Geometry check sheet. Reference: drawing and pictorial views, mm from the part's lowest x, y, z. A direction names the side the tool comes from. Round coordinates to 2 decimals unless told otherwise and drop trailing zeros. Loops run counter-clockwise (first coordinate to the right, second up) from the corner with the lowest first, then second, coordinate; pieces in that order, holes last. Notation, with made-up numbers: (-16.5, 36) - (24.5, 36) arc R18 cw to (24.5, 67) - close; hole circle Ø9 at (16.5, 19). An arc over 180 degrees is marked (long way). Return JSON: item names as keys, results as strings.
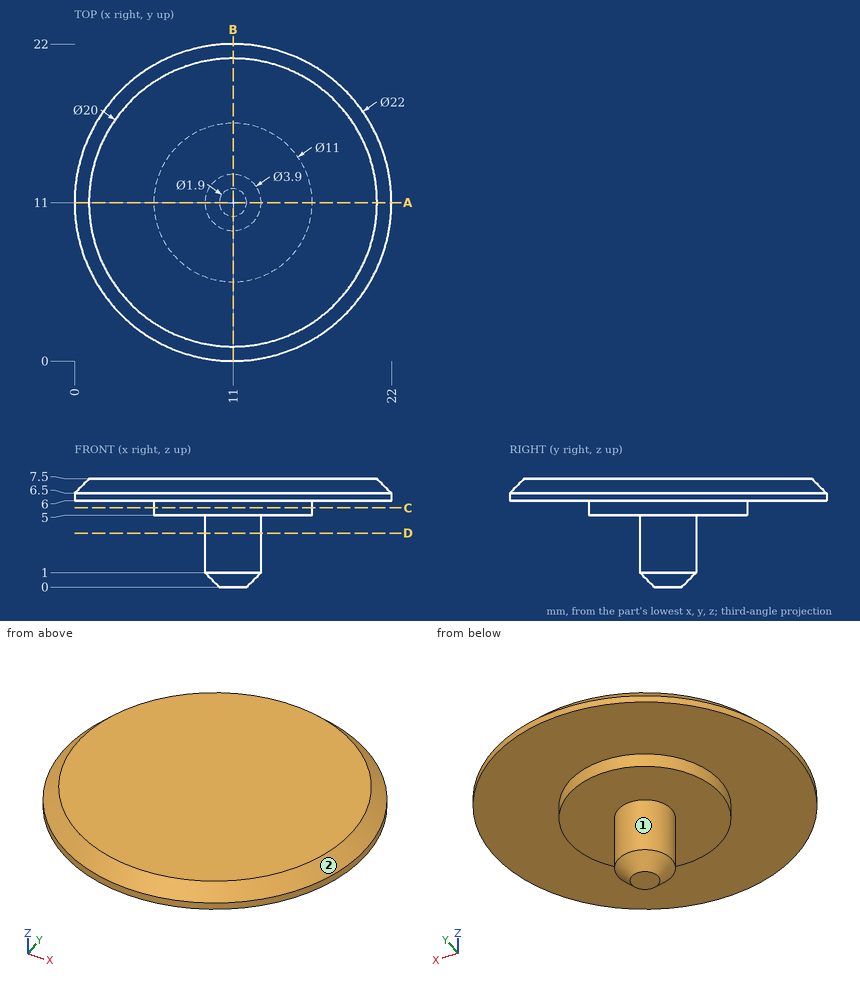
Q1. Sectioned sample at C-C (z = 5.5). Enter the section's corners in (x, y), plus the area to 3 significant figures.
Answer key:
{"outline": "circle Ø11 at (11, 11)", "area": "95.0 mm²"}
Q2. Sectioned sample at A-A (y = 11). Enter the section's corners in (x, z), plus the area to 3 significant figures.
Answer key:
{"outline": "(0, 6) - (5.5, 6) - (5.5, 5) - (9.05, 5) - (9.05, 1) - (10.05, 0) - (11.95, 0) - (12.95, 1) - (12.95, 5) - (16.5, 5) - (16.5, 6) - (22, 6) - (22, 6.5) - (21, 7.5) - (1, 7.5) - (0, 6.5) - close", "area": "61.5 mm²"}
Q3. Tool access check on the marked faces 1 and 2. Record the directions out of +Z, -Z, +X, -X, +Y, -Y that give a thin tool (end or side, any length) a straight path to the whole face; none if there is none.
Answer key:
{"face 1": "-Z", "face 2": "+Z"}
Q4. Sectioned sample at D-D (z = 3.75). Enter the section's corners in (x, y).
Answer key:
{"outline": "circle Ø3.9 at (11, 11)"}
Q5. Depth check by flat-ended pin: P1, Ø1, axis at x = 18.5, y = 4, coming from the -Z side; P2, Ø1.5, axis at y = 6, z = 3, coming from the -X side; P3, Ø6, axis at x = 17.5, y = 15.5, coming from the -Z side. Enter the tip coordinate at first touch or a pass-through.
Answer key:
{"P1": "stops at z = 6", "P2": "passes through", "P3": "stops at z = 5"}
Q6. Scan lines: probe 1 along Z at (x, y) = (7, 15); probe 2 along X at (y, z) = (10.25, 5.5); probe 3 along X at (y, z) = (10.25, 2). Record each from-to range of solid material in increasing order. Write a range as [from, to].
Answer key:
{"probe 1": "z = [6, 7.5]", "probe 2": "x = [5.55, 16.45]", "probe 3": "x = [9.2, 12.8]"}
